The listing builds one solid part. Answer for the finished solid, in the listing's coordinates (mm). A direction names the side the tool comes from. Coordinates: 2 decimals unless noted, no trailing zeros. Order: outer loops, then holes, each group sorted by start corner. A loop starts at its lowest first (then second) coordinate and runs counter-clockwise, first axis right, second up. Notation, with made-up numbers: (62, 88) -> (114, 88) arc R12 cw to (114, 106) -> close; hole circle Ø3 at (17, 71). An arc over 180 degrees is marked (long way). Return JSON: item names as keys, results as strings.
```python
from build123d import *

# Parameters (mm, degrees)
EXTRUDE001_DEPTH = 634
SKETCH020_R      = 2.05
HOLE013_DEPTH    = 1283.986422


with BuildPart() as part:
    # Sketch → Extrude001 (new body)
    with BuildSketch(Plane(origin=(0, 0, 0), x_dir=(0, -1, 0), z_dir=(-1, 0, 0))):
        Polygon((-20, 0), (-20, 15), (0, 15), (0, 13.5), (-18.5, 13.5), (-18.5, 0), align=None)
    extrude(amount=-EXTRUDE001_DEPTH)

    # Sketch020 → Hole013 (cut, through all)
    with BuildSketch(Plane.XY.offset(15)):
        with Locations((6.75, 9.25)):
            Circle(SKETCH020_R)
    hole013 = extrude(amount=-HOLE013_DEPTH, mode=Mode.SUBTRACT)

    # Mirrored007: Hole013 across Sketch020 Axis0
    add(hole013.mirror(Plane(origin=(317, 18.5, 15), x_dir=(0, 0, 1), z_dir=(1, 0, 0))), mode=Mode.SUBTRACT)


with BuildPart() as part_1:
    # Body006 placement: moved
    add(part.part.moved(Location((3, 266.5, 173))))


solid = part_1.part
```
Item 1: The part is cut by section B-B on z = 177.5. Determine the outline of the cut face in (x, y).
Answer list:
{"outline": "(3, 285) -> (637, 285) -> (637, 286.5) -> (3, 286.5) -> close"}
Item 2: Find the intervals of material crossed by probe 1 along X at (y, z) = (275.75, 186.95); probe 2 along Y at (x, z) = (9.75, 187.4); probe 3 along Z at (x, y) = (454, 277), in increasing order.
Answer list:
{"probe 1": "3 to 7.7, 11.8 to 628.2, 632.3 to 637", "probe 2": "266.5 to 273.7, 277.8 to 286.5", "probe 3": "186.5 to 188"}
Item 3: The part is cut by section C-C on y = 281.5. Determine the outline of the cut face in (x, z), plus the area to 3 significant figures.
Answer list:
{"outline": "(3, 186.5) -> (637, 186.5) -> (637, 188) -> (3, 188) -> close", "area": "951 mm2"}
Item 4: The part is cut by section A-A on x = 219.5. Determine the outline of the cut face in (y, z), plus the area to 4 significant figures.
Answer list:
{"outline": "(266.5, 186.5) -> (285, 186.5) -> (285, 173) -> (286.5, 173) -> (286.5, 188) -> (266.5, 188) -> close", "area": "50.25 mm2"}
Item 5: Which of the six approach directions +Z, -Z, +X, -X, +Y, -Y give full straight-line access (tool end or side, diameter ignored) to faces 1 (the flat face through (316, 277, 188)), 2 (the flat face through (316, 285, 180))?
Answer list:
{"face 1": "+Z, +X, -X, +Y, -Y", "face 2": "-Z, +X, -X, -Y"}
Item 6: Flat-ended cylindrical pins translate along their axes: pin 1 (3.5 mm diameter, centred on x = 9.75, y = 275.75, fed in from +Z); pin 2 (8 mm diameter, centred on x = 510.5, y = 275, fed in from -Z); pin 3 (8 mm diameter, centred on x = 533.5, z = 182, fed in from -Y). Find the tip coordinate at first contact, or state that the pin passes through.
Answer list:
{"pin 1": "through", "pin 2": "z = 186.5", "pin 3": "y = 285"}
